from build123d import *

# Parameters (mm, degrees)
EXTRUDE_1_DEPTH     = 3
SKETCH_2_W          = 7.1
SKETCH_2_H          = 5.7
CUT_EXTRUDE_1_DEPTH = 127.757680391
SKETCH_3_R          = 2.05
CUT_EXTRUDE_2_DEPTH = 127.757680391


with BuildPart() as part:
    # 스케치1 → 보스-돌출1 (new body)
    with BuildSketch(Plane.XY):
        with BuildLine():
            Line((77.962543428, 13.364192405), (-57.290239933, 13.364192405))
            Line((-57.290239933, 13.364192405), (-57.290239933, 1.630404544))
            Line((-57.290239933, 1.630404544), (-57.290239933, -6.697716143))
            Line((-57.290239933, -6.697716143), (-57.290239933, -31.635807595))
            Line((-57.290239933, -31.635807595), (102.63413291, -31.635807595))
            ThreePointArc((102.63413291, -31.635807595), (116.82974501, -25.755792538), (122.709760067, -11.560180438))
            Line((122.709760067, -11.560180438), (122.709760067, 2.792586849))
            ThreePointArc((122.709760067, 2.792586849), (119.613408488, 10.267840825), (112.138154512, 13.364192405))
            Line((112.138154512, 13.364192405), (77.962543428, 13.364192405))
        make_face()
    extrude(amount=EXTRUDE_1_DEPTH)

    # 스케치2 → 컷-돌출1 (cut, through all)
    with BuildSketch(Plane(origin=(0, 0, 0), x_dir=(-1, 0, 0), z_dir=(0, 0, -1))):
        with Locations((46.740239933, -28.785807595)):
            Rectangle(SKETCH_2_W, SKETCH_2_H)
    extrude(amount=-CUT_EXTRUDE_1_DEPTH, mode=Mode.SUBTRACT)

    # 스케치3 → 컷-돌출2 (cut, through all)
    with BuildSketch(Plane(origin=(0, 0, 0), x_dir=(-1, 0, 0), z_dir=(0, 0, -1))):
        with Locations((-114.073037193, 3.507033956)):
            Circle(SKETCH_3_R)
        with Locations((-73.198629194, -2.419409625)):
            Circle(SKETCH_3_R)
        with Locations((-114.073037193, -11.492966044)):
            Circle(SKETCH_3_R)
        with Locations((-13.198629194, -2.419409625)):
            Circle(SKETCH_3_R)
    extrude(amount=-CUT_EXTRUDE_2_DEPTH, mode=Mode.SUBTRACT)


solid = part.part
Design review of the part built by this model. Coordinates are the model's own, in mm. A direction names the side the tool comes from. Coordinates: 2 decimals unless noted, no trailing zeros. Loops run counter-clockwise (first coordinate to the right, second up) from the corner with the lowest first, then second, coordinate; pieces in that order, holes last. Notation, with made-up numbers: (42, -10.5) -> (88, -10.5) arc R26 ccw to (88, 7.5) -> close; hole circle Ø9 at (83.25, -10.5). An arc over 180 degrees is marked (long way). Use a Markdown table: item, result. Add a question column.
Item 1: Wall thickness on L1, parallel to Y at x = 114, z = 1.6; L2, parallel to Y at x = -43.5, z = 0.5; L3, parallel to X at y = -12.5, z = 0.7: over which ranges is each line inside the solid? List them lowest first. Write a range as from..to.
Item 2: We need section B-B, the plane y = -22.5. Write out the cut boundary in (x, z).
Item 3: We need section A-A, the plane z = 2.5. Write out the cut boundary in (x, y).
Item 4: The part is to be moulded in two halves that separate along X. For faces 3 (the flat face through (31, -9, 0)), 4 (the flat face through (-57.29, -9, 1)), 5 (the cylindrical face through (15.247, -2.329, 1.479)), say which applies: +X half, -X half, draft (parallel to the pull), parting line (faces both ways), or undercut.
Item 5: Machinability: for faces 1 (the flat face through (-43.19, -29, 1)), 2 (the flat face through (29, -31.636, 1)), which of the approach directions +Z, -Z, +X, -X, +Y, -Y give a long, thin tool a straight path to every point of the face, cutting with its end or side? Answer none if there is none.
Numbers:
| question | item | result |
|---|---|---|
| 1 | L1 | y = -28.11..-13.54, -9.44..1.46, 5.56..13.2 |
| 1 | L2 | y = -25.94..13.36 |
| 1 | L3 | x = -57.29..112.29, 115.86..122.69 |
| 2 | outline | (-57.29, 0) -> (119.47, 0) -> (119.47, 3) -> (-57.29, 3) -> close |
| 3 | outline | (-57.29, -31.64) -> (-50.29, -31.64) -> (-50.29, -25.94) -> (-43.19, -25.94) -> (-43.19, -31.64) -> (102.63, -31.64) arc R20.08 ccw to (122.71, -11.56) -> (122.71, 2.79) arc R10.57 ccw to (112.14, 13.36) -> (-57.29, 13.36) -> close; hole circle Ø4.1 at (13.2, -2.42); hole circle Ø4.1 at (73.2, -2.42); hole circle Ø4.1 at (114.07, -11.49); hole circle Ø4.1 at (114.07, 3.51) |
| 4 | face 3 | draft |
| 4 | face 4 | -X half |
| 4 | face 5 | undercut |
| 5 | face 1 | +Z, -Z, -Y |
| 5 | face 2 | +Z, -Z, +X, -X, -Y |
